Read the model definition and answer for the solid it produces. Units are mm, in the model's axes. A direction names the side the tool comes from. Give positions to 0.01 mm unless a question says otherwise; leave off trailing zeros. Order: outer loops, then holes, each group sorted by start corner. A loop starts at its lowest first (then second) coordinate and runs counter-clockwise, first axis right, second up. Notation, with made-up numbers: (85, 50.25) - (143, 50.25) arc R21 ccw to (143, 63.25) - close; hole circle Ø5 at (4.25, 2). An arc over 180 degrees is marked (long way). Return JSON: item names as keys, results as strings.
Autodesk Inventor part; units mm, degrees
ref_plane "YZ Plane" through (0, 0, 0) normal (1, 0, 0) x (0, 1, 0)
ref_plane "XZ Plane" through (0, 0, 0) normal (0, 1, 0) x (-1, 0, 0)
ref_plane "XY Plane" through (0, 0, 0) normal (0, 0, 1) x (1, 0, 0)
sketch "スケッチ1" plane through (0, 0, 0) normal (0, 0, 1) x (1, 0, 0)
  circle A0 centre (0, 0) radius 3.45
  dimension "d0" = 6.9
extrude "押し出し1" add sketch "スケッチ1" along normal blind 4
sketch "スケッチ2" plane through (0, 0, 0) normal (0, 0, -1) x (-1, 0, 0)
  circle A0 centre (0, 0) radius 2
  dimension "d3" = 4
extrude "押し出し2" add sketch "スケッチ2" along normal blind 5
thread "ねじ1"
chamfer "面取り1" distance 0.4 angle 45 1 edges at (-3.45, 0, 4)
properties part number "M4×5" material "ステンレス鋼"
Q1. A cutting plane is placed at A-A (x = 0). Write down the section's boundary in (y, z).
Values:
{"outline": "(-3.45, 0) - (-2, 0) - (-2, -5) - (2, -5) - (2, 0) - (3.45, 0) - (3.45, 3.6) - (3.05, 4) - (-3.05, 4) - (-3.45, 3.6) - close"}
Q2. Consider L1, parallel to Z at x = 2.75, y = -0.75; L2, parallel to Y at x = 0.5, z = -2.5; L3, parallel to Y at x = -1, z = -0.75. Determine where each line is inside the solid, lowest interval first.
Values:
{"L1": "z = 0 to 4", "L2": "y = -1.94 to 1.94", "L3": "y = -1.73 to 1.73"}
Q3. A cutting plane is placed at B-B (z = 3.25). Write down the section's boundary in (x, y).
Values:
{"outline": "circle Ø6.9 at (0, 0)"}
Q4. Given pin 1 (4 mm diameter, centred on x = 2.5, z = 1.5, fed in from -Y); pin 2 (2 mm diameter, centred on x = 2, y = -2.5, fed in from -Z); pin 3 (1 mm diameter, centred on x = -2.5, z = 0.5, fed in from -Y), each flat-ended and moving along its own axis, determine where each tip first touches the part or whether it passes through.
Values:
{"pin 1": "stops at y = -3.41", "pin 2": "stops at z = 0", "pin 3": "stops at y = -2.81"}
Q5. A cutting plane is placed at C-C (z = -3.5). Write down the section's boundary in (x, y).
Values:
{"outline": "circle Ø4 at (0, 0)"}
Q6. For faces 1 (the cylindrical face through (-0.45, -3.42, 1.77)), 2 (the cylindrical face through (0, 2, -2)), determine the directions among +Z, -Z, +X, -X, +Y, -Y from which every point of the face is accessible in a straight line to the end or side of a thin tool.
Values:
{"face 1": "+Z, -Z", "face 2": "-Z"}
